Model file for the job. Use its own axes, mm. Face numbers are marked on the shaded views. A direction names the side the tool comes from. Coordinates: 2 decimals unless noted, no trailing zeros. Order: outer loops, then holes, each group sorted by start corner. A loop starts at its lowest first (then second) coordinate and runs counter-clockwise, first axis right, second up. Notation, with made-up numbers: (48, -25) - (94, -25) arc R11 cw to (94, -18) - close; hole circle Ø3 at (30, 6). An arc over 180 degrees is marked (long way). Put each result on its own line as item: value. Start each with the question number.
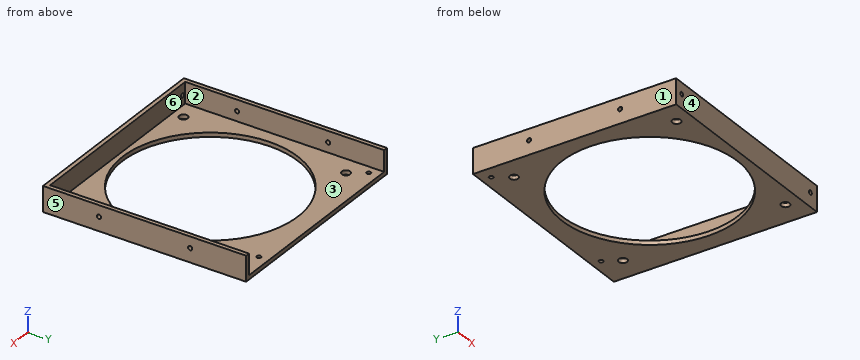
```python
from build123d import *

# Parameters (mm, degrees)
F0_W     = 3
F0_H     = 142
F0_W_2   = 144
F0_R     = 3
F0_R_2   = 62.5
F0_R_3   = 1.5
F0_H_2   = 3
F1_DEPTH = 3
F2_DEPTH = 15
F5_R     = 1.5
F6_DEPTH = 3
F4_R     = 1.5
F7_DEPTH = 25
F3_R     = 1.5
F8_DEPTH = 25


with BuildPart() as f1:
    # F0 (on Top) → F1 (new body)
    with BuildSketch(Plane.XY):
        with Locations((-57.4185222983, 8.8288192153)):
            Rectangle(F0_W, F0_H)
        with Locations((16.0814777017, 8.8288192153)):
            Rectangle(F0_W_2, F0_H)
        with Locations((-42.3870939074, -54.3524108875)):
            Circle(F0_R, mode=Mode.SUBTRACT)
        with Locations((73.6129060926, -54.3524108875)):
            Circle(F0_R, mode=Mode.SUBTRACT)
        with Locations((15.6129060926, 3.6475891125)):
            Circle(F0_R_2, mode=Mode.SUBTRACT)
        with Locations((-42.3870939074, 61.6475891125)):
            Circle(F0_R, mode=Mode.SUBTRACT)
        with Locations((-49.9185222983, 72.8288192153)):
            Circle(F0_R_3, mode=Mode.SUBTRACT)
        with Locations((73.6129060926, 61.6475891125)):
            Circle(F0_R, mode=Mode.SUBTRACT)
        with Locations((67.0814777017, 72.8288192153)):
            Circle(F0_R_3, mode=Mode.SUBTRACT)
        with Locations((89.5814777017, 8.8288192153)):
            Rectangle(F0_W, F0_H)
        with Locations((16.0814777017, -63.6711807847)):
            Rectangle(F0_W_2, F0_H_2)
        with Locations((89.5814777017, -63.6711807847)):
            Rectangle(F0_W, F0_H_2)
        with Locations((-57.4185222983, -63.6711807847)):
            Rectangle(F0_W, F0_H_2)
    extrude(amount=-F1_DEPTH)

    # F0 (on Top) → F2 (join)
    with BuildSketch(Plane.XY):
        with Locations((-57.4185222983, 8.8288192153)):
            Rectangle(F0_W, F0_H)
        with Locations((-57.4185222983, -63.6711807847)):
            Rectangle(F0_W, F0_H_2)
        with Locations((16.0814777017, -63.6711807847)):
            Rectangle(F0_W_2, F0_H_2)
        with Locations((89.5814777017, -63.6711807847)):
            Rectangle(F0_W, F0_H_2)
        with Locations((89.5814777017, 8.8288192153)):
            Rectangle(F0_W, F0_H)
    extrude(amount=F2_DEPTH)

    # F5 (on face) → F6 (cut)
    with BuildSketch(Plane(origin=(-58.9185222983, 0, 0), x_dir=(0, -1, 0), z_dir=(-1, 0, 0))):
        with Locations((25.1711807847, 7)):
            Circle(F5_R)
        with Locations((-39.8288192153, 7)):
            Circle(F5_R)
    extrude(amount=-F6_DEPTH, mode=Mode.SUBTRACT)

    # F4 (on face) → F7 (cut)
    with BuildSketch(Plane.XZ.offset(65.1711807847)):
        with Locations((-52.9185222983, 7)):
            Circle(F4_R)
        with Locations((84.0814777017, 7)):
            Circle(F4_R)
    extrude(amount=-F7_DEPTH, mode=Mode.SUBTRACT)

    # F3 (on face) → F8 (cut)
    with BuildSketch(Plane.YZ.offset(91.0814777017)):
        with Locations((-25.1711807847, 7)):
            Circle(F3_R)
        with Locations((39.8288192153, 7)):
            Circle(F3_R)
    extrude(amount=-F8_DEPTH, mode=Mode.SUBTRACT)


solid = f1.part
```
Item 1: 3-axis set-ups, long thin cutter, end or side, ignore diameter. For the marked faces 5 and 6: which of +Z, -Z, +X, -X, +Y, -Y reach the whole face in a straight line?
Item 2: Wall check: line 1 along X through (y, z) = (-43, 7.5); line 2 along Z through (x, y) = (35, 72); line 3 along Y through (x, z) = (67, 10). Give the ranges that are in metal, low to high.
Item 3: Slice it at A-A, the plane x = -21. Give the cut face in (y, z).
Item 4: Flat gauge pins, fed straight in: pin 1 Ø10 at (x, y) = (63.5, -31) entering from +Z; pin 2 Ø3.5 at (x, y) = (67.08, 72.83) entering from -Z; pin 3 Ø5 at (x, z) = (-52.92, 7) entering from +Y. Where does each tip first touch, or does it go through?
Item 5: Pull direction X, two halves, no side cores. Call the marked faces 1, 2, 3 and 4: pulls with the +X half, pulls with the -X half, needs draft (parallel to the pull), parting line crosses it, or undercut.
Item 6: Slice it at D-D, the plane x = 73.5. Give the cut face in (y, z), plus the area to 3 significant figures.
Item 7: Slice it at C-C, the plane z = 11.25. Give the cut face in (x, y).
Item 8: Slice it at B-B, the plane y = -39. Give the cut face in (x, z), plus the area to 3 significant figures.
Here are the results:
1. face 5: +Z, -Z, +X, +Y, -Y
1. face 6: +Z, +Y
2. line 1: x = -58.92 to -55.92, 88.08 to 91.08
2. line 2: z = -3 to 0
2. line 3: y = -65.17 to -62.17
3. outline: (-65.17, -3) - (-47.01, -3) - (-47.01, 0) - (-62.17, 0) - (-62.17, 15) - (-65.17, 15) - close; (54.3, -3) - (79.83, -3) - (79.83, 0) - (54.3, 0) - close
4. pin 1: stops at z = 0
4. pin 2: stops at z = -3
4. pin 3: stops at y = -62.17
5. face 1: pulls with the -X half
5. face 2: undercut
5. face 3: undercut
5. face 4: needs draft
6. outline: (-65.17, -3) - (-57.35, -3) - (-57.35, 0) - (-62.17, 0) - (-62.17, 15) - (-65.17, 15) - close; (-51.35, -3) - (-19.92, -3) - (-19.92, 0) - (-51.35, 0) - close; (27.21, -3) - (58.65, -3) - (58.65, 0) - (27.21, 0) - close; (64.65, -3) - (79.83, -3) - (79.83, 0) - (64.65, 0) - close
6. area: 303 mm^2
7. outline: (-58.92, -65.17) - (91.08, -65.17) - (91.08, 79.83) - (88.08, 79.83) - (88.08, -62.17) - (-55.92, -62.17) - (-55.92, 79.83) - (-58.92, 79.83) - close
8. outline: (-58.92, -3) - (-30.08, -3) - (-30.08, 0) - (-55.92, 0) - (-55.92, 15) - (-58.92, 15) - close; (61.3, -3) - (91.08, -3) - (91.08, 15) - (88.08, 15) - (88.08, 0) - (61.3, 0) - close
8. area: 266 mm^2
